Source: CAD feature listing. Evaluate the final solid. Frame: model axes, mm. Face numbers are marked on the shaded views. A direction names the side the tool comes from. Give positions to 0.01 mm unless a question says otherwise; leave off trailing zeros. Loops run counter-clockwise (first coordinate to the right, second up) from the corner with the lowest first, then second, coordinate; pieces in that order, holes last. Notation, with made-up numbers: M 23.5,-10 L 82.5,-10 A9 cw 82.5,-4 Z; hole C 50,34 d8. An arc over 180 degrees is marked long. Answer in a Markdown table with one row per item.
```python
from build123d import *

# Parameters (mm, degrees)
SKETCH2_R           = 10
BOSS_EXTRUDE1_DEPTH = 50
SKETCH3_W           = 40
SKETCH3_H           = 50
CUT_EXTRUDE1_DEPTH  = 55
SKETCH4_R           = 5
BOSS_EXTRUDE2_DEPTH = 48
SKETCH5_R           = 2.5
CUT_EXTRUDE2_DEPTH  = 10


with BuildPart() as part:
    # Sketch2 → Boss-Extrude1 (new body)
    with BuildSketch(Plane.XY):
        with BuildLine():
            Line((15, 0), (15, -35))
            Line((15, -35), (-15, -35))
            Line((-15, -35), (-15, 0))
            ThreePointArc((-15, 0), (0, 15), (15, 0))
        make_face()
        Circle(SKETCH2_R, mode=Mode.SUBTRACT)
    extrude(amount=-BOSS_EXTRUDE1_DEPTH)

    # Sketch3 → Cut-Extrude1 (cut)
    with BuildSketch(Plane(origin=(15, 0, 0), x_dir=(0, 0, -1), z_dir=(1, 0, 0))):
        with Locations((25, -10)):
            Rectangle(SKETCH3_W, SKETCH3_H)
    extrude(amount=-CUT_EXTRUDE1_DEPTH, mode=Mode.SUBTRACT)


with BuildPart() as cut_extrude1_piece_1:
    # of the separate pieces the step leaves, piece 1, a body of its own (cut_extrude1_pieces)
    add(part.part.solids().sort_by_distance((15, 0, 0))[0])



with BuildPart() as cut_extrude1_piece_2:
    # of the separate pieces the step leaves, piece 2, a body of its own (cut_extrude1_pieces)
    add(part.part.solids().sort_by_distance((15, 0, -45))[0])


with BuildPart() as cut_extrude1_piece_1_1:
    add(cut_extrude1_piece_1.part)

    add(cut_extrude1_piece_2.part)  # Boss-Extrude2 merges Cut-Extrude1 piece 2
    # Sketch4 → Boss-Extrude2 (add)
    with BuildSketch(Plane(origin=(0, 0, -50), x_dir=(-1, 0, 0), z_dir=(0, 0, -1))):
        with Locations((0, -29)):
            Circle(SKETCH4_R)
    extrude(amount=-BOSS_EXTRUDE2_DEPTH)

    # Sketch5 → Cut-Extrude2 (cut, symmetric)
    with BuildSketch(Plane(origin=(0, 0, 0), x_dir=(0, 0, -1), z_dir=(1, 0, 0))):
        with Locations((25, -29)):
            Circle(SKETCH5_R)
    extrude(amount=CUT_EXTRUDE2_DEPTH, both=True, mode=Mode.SUBTRACT)


solid = cut_extrude1_piece_1_1.part
```
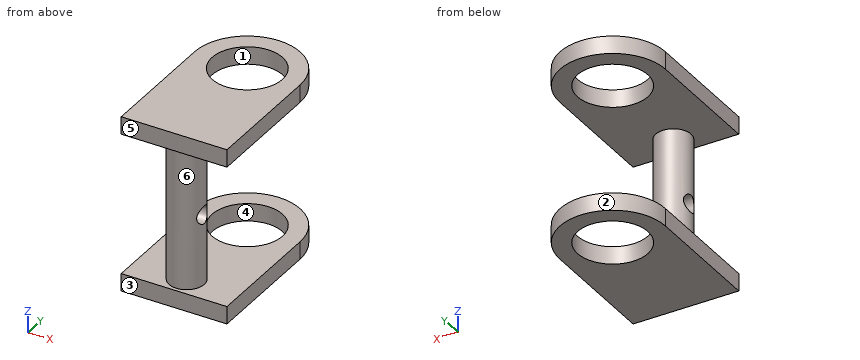
1) Section A-A, the plane y = -8. Return loops of the section in (x, z).
Reply:
| item | result |
|---|---|
| outline | M -15,-50 L -6,-50 L -6,-45 L -15,-45 Z; M -15,-5 L -6,-5 L -6,0 L -15,0 Z; M 6,-50 L 15,-50 L 15,-45 L 6,-45 Z; M 6,-5 L 15,-5 L 15,0 L 6,0 Z |
2) Set-up query: the marked faces 5 and 6. Return all of +Z, -Z, +X, -X, +Y, -Y with unobstructed straight access to the full face (end or side cutting, diameter ignored); none if empty.
Reply:
| item | result |
|---|---|
| face 5 | +Z, -Z, +X, -X, -Y |
| face 6 | none |
3) Section D-D, the plane x = -9. Return loops of the section in (y, z), then the cut area to 3 significant figures.
Reply:
| item | result |
|---|---|
| outline | M -35,-50 L -4.36,-50 L -4.36,-45 L -35,-45 Z; M -35,-5 L -4.36,-5 L -4.36,0 L -35,0 Z; M 4.36,-50 L 12,-50 L 12,-45 L 4.36,-45 Z; M 4.36,-5 L 12,-5 L 12,0 L 4.36,0 Z |
| area | 383 mm² |
4) Section B-B, the plane x = 0. Return loops of the section in (y, z).
Reply:
| item | result |
|---|---|
| outline | M -35,-50 L -10,-50 L -10,-45 L -24,-45 L -24,-5 L -10,-5 L -10,0 L -35,0 L -35,-5 L -34,-5 L -34,-45 L -35,-45 Z; M 10,-50 L 15,-50 L 15,-45 L 10,-45 Z; M 10,-5 L 15,-5 L 15,0 L 10,0 Z; hole C -29,-25 d5 |
5) Pin query (flat end, axial travel): pin 1 Ø15 at (x, y) = (-3.5, -21.5) entering from +Z; pin 2 Ø6 at (y, z) = (-29, -25) entering from -X; pin 3 Ø5 at (x, z) = (-5.5, -30) entering from +Y; pin 4 Ø1 at (x, z) = (-5, -7.5) entering from +Y. Return the tip coordinate at first contact, or that it passes through.
Reply:
| item | result |
|---|---|
| pin 1 | stops at z = 0 |
| pin 2 | stops at x = -5 |
| pin 3 | stops at y = -25 |
| pin 4 | stops at y = -26.82 |
6) Pull-direction query (X, two-part tool) for the marked faces 1, 2, 3 and 4; classes: released by +X, released by -X, zero draft, split by the parting line, or undercut.
Reply:
| item | result |
|---|---|
| face 1 | undercut |
| face 2 | split by the parting line |
| face 3 | zero draft |
| face 4 | undercut |
7) Material intervals for L1, parallel to Z at x = 1, y = 10; L2, parallel to Z at x = -2, y = -29; L3, parallel to Y at x = 0, z = -1.75, sorted ascending.
Reply:
| item | result |
|---|---|
| L1 | z = -50 to -45, -5 to 0 |
| L2 | z = -50 to -27.5, -22.5 to 0 |
| L3 | y = -35 to -10, 10 to 15 |
8) Section C-C, the plane y = -29. Return loops of the section in (x, z).
Reply:
| item | result |
|---|---|
| outline | M -15,-50 L 15,-50 L 15,-45 L 5,-45 L 5,-27.5 L -5,-27.5 L -5,-45 L -15,-45 Z; M -15,-5 L -5,-5 L -5,-22.5 L 5,-22.5 L 5,-5 L 15,-5 L 15,0 L -15,0 Z |
